from build123d import *

# Parameters (mm, degrees)
F0_R     = 38.1
F0_R_2   = 1.5
F0_R_3   = 31.75
F1_DEPTH = 127
F2_R     = 6
F3_DEPTH = 42.2
F4_R     = 1.5
F5_DEPTH = 10
F6_COUNT = 4
F7_DEPTH = 20
F8_COUNT = 4


with BuildPart() as f1:
    # F0 (on Top) → F1 (new body)
    with BuildSketch(Plane.XY):
        Circle(F0_R)
        with Locations((0, -35)):
            Circle(F0_R_2, mode=Mode.SUBTRACT)
        Circle(F0_R_3, mode=Mode.SUBTRACT)
        with Locations((0, -35)):
            Circle(F0_R_2)
    extrude(amount=F1_DEPTH)

    # F2 (on Front) → F3 (cut)
    with BuildSketch(Plane.XZ):
        with Locations((0, 50)):
            Circle(F2_R)
    extrude(amount=-F3_DEPTH, mode=Mode.SUBTRACT)

    # F6: F5 ×4 about axis
    f6_axis = Axis((0, 0, 127), (0, 0, 1))


with BuildPart() as f5:
    # F4 (on face) → F5 (new body)
    with BuildSketch(Plane.XY.offset(127)):
        with Locations((0, 35)):
            Circle(F4_R)
    extrude(amount=-F5_DEPTH)


with BuildPart() as f1_1:
    add(f1.part)
    for i in range(1, F6_COUNT):
        add(f5.part.rotate(f6_axis, i * 360 / F6_COUNT), mode=Mode.SUBTRACT)

    # F6#seed: cut F5
    add(f5.part, mode=Mode.SUBTRACT)

    # F8: F7 ×4 about axis
    f8_axis = Axis((0, 0, 0), (0, 0, 1))


with BuildPart() as f7:
    # F0 (on Top) → F7 (new body)
    with BuildSketch(Plane.XY):
        with Locations((0, -35)):
            Circle(F0_R_2)
    extrude(amount=F7_DEPTH)


with BuildPart() as f1_2:
    add(f1_1.part)
    for i in range(1, F8_COUNT):
        add(f7.part.rotate(f8_axis, i * 360 / F8_COUNT), mode=Mode.SUBTRACT)

    # F8#seed: cut F7
    add(f7.part, mode=Mode.SUBTRACT)


solid = f1_2.part
Model file for the job. Use its own axes, mm. A direction names the side the tool comes from. Round coordinates to 2 decimals unless told otherwise and drop trailing zeros. Loops run counter-clockwise (first coordinate to the right, second up) from the corner with the lowest first, then second, coordinate; pieces in that order, holes last. Notation, with made-up numbers: (-6, -9) -> (15, -9) arc R21 ccw to (15, 12) -> close; hole circle Ø3 at (9.25, -2.5). An arc over 180 degrees is marked (long way). Answer as CSV lines item,"result". Start each with the question number.
1) Mould opens along X. For faces 1 (the face through (-8.259, -37.194, 62.611)), 2 (the face through (-36.464, 0.325, 9.86)), 3 (the face through (-23, 23, 0)) say: +X half, -X half, draft (parallel to the pull), parting line (faces both ways), or undercut.
2) Slice it at B-B (x = 0). List the corners of the cut face in (y, z), plus the area to 3 significant figures.
3) Pin check, flat tips, straight feed: P1, Ø1, axis at y = -18, z = 81, coming from the +X side; P2, Ø1, axis at x = -14.5, z = 24.5, coming from the +Y side; P3, Ø2.5, axis at x = 35, y = 0, coming from the -Z side. Stop position of each tip, or through.
4) Probe line 1 along Y through (x, z) = (0, 6.25); line 2 along Y through (x, z) = (0.5, 90); line 3 along X through (y, z) = (-7.5, 77.5). List the from-to ranges inside material, lowest first.
5) Slice it at D-D (x = -13). List the corners of the cut face in (y, z).
6) Slice it at A-A (y = 0). List the corners of the cut face in (x, z).
7) Slice it at C-C (z = 11). List the corners of the cut face in (x, y).
8) Tool access for faces 4 (the face through (35, 0, 20)), 5 (the face through (-4.76, 34.59, 46.35)), 6 (the face through (33.536, 0.325, 122.07)): list every direction of +Z, -Z, +X, -X, +Y, -Y with a clear straight run to the whole face (end or side of a thin tool).
Filled in:
1,face 1,"parting line"
1,face 2,"undercut"
1,face 3,"draft"
2,outline,"(-38.1, 0) -> (-36.5, 0) -> (-36.5, 20) -> (-33.5, 20) -> (-33.5, 0) -> (-31.75, 0) -> (-31.75, 127) -> (-33.5, 127) -> (-33.5, 117) -> (-36.5, 117) -> (-36.5, 127) -> (-38.1, 127) -> close; (31.75, 0) -> (33.5, 0) -> (33.5, 20) -> (36.5, 20) -> (36.5, 0) -> (38.1, 0) -> (38.1, 44) -> (31.75, 44) -> close; (31.75, 56) -> (38.1, 56) -> (38.1, 127) -> (36.5, 127) -> (36.5, 117) -> (33.5, 117) -> (33.5, 127) -> (31.75, 127) -> close"
2,area,"1,360 mm2"
3,P1,"stops at x = 33.84"
3,P2,"stops at y = 35.43"
3,P3,"stops at z = 20"
4,line 1,"y = -38.1 to -36.5, -33.5 to -31.75, 31.75 to 33.5, 36.5 to 38.1"
4,line 2,"y = -38.1 to -31.75, 31.75 to 38.1"
4,line 3,"x = -37.35 to -30.85, 30.85 to 37.35"
5,outline,"(-35.81, 0) -> (-28.97, 0) -> (-28.97, 127) -> (-35.81, 127) -> close; (28.97, 0) -> (35.81, 0) -> (35.81, 127) -> (28.97, 127) -> close"
6,outline,"(-38.1, 0) -> (-36.5, 0) -> (-36.5, 20) -> (-33.5, 20) -> (-33.5, 0) -> (-31.75, 0) -> (-31.75, 127) -> (-33.5, 127) -> (-33.5, 117) -> (-36.5, 117) -> (-36.5, 127) -> (-38.1, 127) -> close; (31.75, 0) -> (33.5, 0) -> (33.5, 20) -> (36.5, 20) -> (36.5, 0) -> (38.1, 0) -> (38.1, 127) -> (36.5, 127) -> (36.5, 117) -> (33.5, 117) -> (33.5, 127) -> (31.75, 127) -> close"
7,outline,"circle Ø76.2 at (0, 0); hole circle Ø3 at (-35, 0); hole circle Ø63.5 at (0, 0); hole circle Ø3 at (0, -35); hole circle Ø3 at (0, 35); hole circle Ø3 at (35, 0)"
8,face 4,"-Z"
8,face 5,"+Y"
8,face 6,"+Z"
